CAD build for the part. Positions are in the model's coordinates, mm. A direction names the side the tool comes from. Give positions to 0.01 mm unless a question says otherwise; leave off trailing zeros. Write each loop counter-clockwise with the first axis right and the second up, starting at its lowest first coordinate (ties: lowest second). Pieces come first, ordered by that corner, then holes. Notation, with made-up numbers: (62.5, 27) - (80.5, 27) arc R26 cw to (80.5, 53) - close; hole circle Ø1 at (-27, 51.5). An arc over 180 degrees is marked (long way). Answer as a JSON object with one key per item and string values.
from build123d import *

# Parameters (mm, degrees)
SKETCH1_W                          = 38.1
SKETCH1_H                          = 47.625
BOSS_EXTRUDE1_DEPTH                = 19.05
CUT_EXTRUDE1_REACH                 = 21.05
SKETCH2_W                          = 19.05
SKETCH2_H                          = 28.575
F_5_16_24_TAPPED_HOLE1_D           = 6.9088
F_5_16_24_TAPPED_HOLE1_DEPTH       = 19.06
F_5_16_24_TAPPED_HOLE1_CSINK_D     = 9.2075
F_5_16_24_TAPPED_HOLE1_CSINK_ANGLE = 90
F_5_16_24_TAPPED_HOLE1_TIP         = 2.075612922
F_5_16_CLEARANCE_HOLE1_D           = 8.2042
F_5_16_CLEARANCE_HOLE1_CSINK_D     = 9.4742
F_5_16_CLEARANCE_HOLE1_CSINK_ANGLE = 90
CHAMFER1_SIZE                      = 1.5


with BuildPart() as part:
    # Sketch1 → Boss-Extrude1 (new body)
    with BuildSketch(Plane(origin=(0, 0, 0), x_dir=(1, 0, 0), z_dir=(0, 1, 0))):
        Rectangle(SKETCH1_W, SKETCH1_H)
    extrude(amount=BOSS_EXTRUDE1_DEPTH)

    # Sketch2 → Cut-Extrude1 (cut, up to next)
    with BuildSketch(Plane(origin=(0, 19.05, 0), x_dir=(1, 0, 0), z_dir=(0, 1, 0)), mode=Mode.PRIVATE) as cut_extrude1_sk1:
        with Locations((9.525, 9.525)):
            Rectangle(SKETCH2_W, SKETCH2_H)
    cut_extrude1_tool1 = extrude(cut_extrude1_sk1.sketch, amount=-CUT_EXTRUDE1_REACH, mode=Mode.PRIVATE) & part.part
    add(cut_extrude1_tool1.solids().sort_by_distance((9.525, 19.05, -9.525))[0], mode=Mode.SUBTRACT)

    # 5/16-24 Tapped Hole1
    with Locations(Plane.ZY.offset(19.05)):
        with Locations((-14.2875, 9.525), (11.1125, 9.525)):
            CounterSinkHole(F_5_16_24_TAPPED_HOLE1_D / 2, F_5_16_24_TAPPED_HOLE1_CSINK_D / 2, depth=F_5_16_24_TAPPED_HOLE1_DEPTH, counter_sink_angle=F_5_16_24_TAPPED_HOLE1_CSINK_ANGLE)
            with Locations((0, 0, -(F_5_16_24_TAPPED_HOLE1_DEPTH + F_5_16_24_TAPPED_HOLE1_TIP / 2))):  # 118° drill point
                Cone(0, F_5_16_24_TAPPED_HOLE1_D / 2, F_5_16_24_TAPPED_HOLE1_TIP, mode=Mode.SUBTRACT)

    # 5/16 Clearance Hole1 (through all)
    with Locations(Plane(origin=(0, 0, 4.7625), x_dir=(-1, 0, 0), z_dir=(0, 0, -1))):
        with Locations((-9.525, 9.525)):
            CounterSinkHole(F_5_16_CLEARANCE_HOLE1_D / 2, F_5_16_CLEARANCE_HOLE1_CSINK_D / 2, counter_sink_angle=F_5_16_CLEARANCE_HOLE1_CSINK_ANGLE)

    # Chamfer1
    chamfer1_edges = [part.edges().sort_by_distance(p)[0] for p in [
        (-9.525, 0, -23.8125),
        (-9.525, 19.05, -23.8125),
        (9.525, 0, 4.7625),
        (19.05, 9.525, 4.7625),
        (0, 9.525, -23.8125),
        (9.525, 19.05, 4.7625),
    ]]
    chamfer(chamfer1_edges, length=CHAMFER1_SIZE)


solid = part.part
Item 1: Cut at C-C (z = 3). Give the cut face in (x, y).
Entries:
{"outline": "(-19.05, 0) - (0, 0) - (0, 19.05) - (-19.05, 19.05) - close"}
Item 2: Probe line 1 (Z direction, x = -6, y = 11.25); line 2 (X direction, y = 2.75, z = -8); line 3 (Z direction, x = 16, y = 17.5). List the from-to ranges inside material, lowest first. Write a range as from..to.
Entries:
{"line 1": "-23.81..-17.28, -11.29..8.12, 14.11..23.81", "line 2": "-19.05..0", "line 3": "4.76..23.81"}
Item 3: Cut at D-D (x = 16). Give the cut face in (y, z), and give its area (3 significant figures).
Entries:
{"outline": "(0, 6.26) - (1.5, 4.76) - (17.55, 4.76) - (19.05, 6.26) - (19.05, 23.81) - (0, 23.81) - close", "area": "361 mm2"}
Item 4: Which spindle directions (+Z, -Z, +X, -X, +Y, -Y) get a long thin tool onto all of the face, cutting with end or side? Do faces 1 (the flat face through (9.39, 18.31, 5.52)), 2 (the flat face through (9.66, 0.74, 5.52)), 3 (the cylindrical face through (-8.82, 11.86, 13.66)), 4 (the flat face through (-0.76, 9.66, -23.07)). Say none if no direction does.
Entries:
{"face 1": "-Z, +X, +Y", "face 2": "-Z, +X, -Y", "face 3": "-X", "face 4": "-Z, +X, +Y, -Y"}
Item 5: Cut at A-A (x = -6.5). State how many separate pieces and enclosed holes the cut face has, and give its area (3 significant figures).
Entries:
{"separate pieces": "1", "enclosed holes": "2", "area": "830 mm2"}
Item 6: Flat gauge pins, fed straight in: P1, Ø8, axis at y = 9.52, z = 11.11, coming from the -X side; P2, Ø1, axis at x = 8.5, y = 16, coming from the -Z side. Where does each tip first touch, or does it go through?
Entries:
{"P1": "x = -18.45", "P2": "z = 4.76"}
Item 7: Cut at B-B (y = 15.75). Give the cut face in (x, z), and give its area (3 significant figures).
Entries:
{"outline": "(-19.05, -23.81) - (-1.5, -23.81) - (0, -22.31) - (0, 4.76) - (17.55, 4.76) - (19.05, 6.26) - (19.05, 23.81) - (-19.05, 23.81) - close", "area": "1,270 mm2"}
Item 8: Mould opens along Z. For faces 5 (the cylindrical face through (-8.825, 10.563, -17.582)), 6 (the flat face through (-5, 19.05, 6)), 7 (the flat face through (0, 9, 23.812)) say: +Z half, -Z half, draft (parallel to the pull), parting line (faces both ways), or undercut.
Entries:
{"face 5": "undercut", "face 6": "draft", "face 7": "+Z half"}
